For this review, take the finished solid that the model builds, in its own axes (mm). Face numbers are marked on the shaded views. A direction names the side the tool comes from. Coordinates: 2 decimals unless noted, no trailing zeros. Loops run counter-clockwise (first coordinate to the right, second up) from the corner with the lowest first, then second, coordinate; pieces in that order, holes last.
1. Take a section at A-A, the plane x = 23. State the section outline as (y, z) points, then the cut area to 3 significant figures.
2. Take a section at C-C, the plane y = 8. State the section outline as (x, z) points.
3. Machinability: for the marked faces 1, 2 and 3, which of the approach directions +Z, -Z, +X, -X, +Y, -Y give a long, thin tool a straight path to every point of the face, cutting with its end or side? Answer none if there is none.
4. Clearance check with flat-ended pins moving along their axes: P1, Ø1, axis at y = 19, z = 10, coming from the -X side; P2, Ø5.5, axis at x = -25, z = 7.5, coming from the +Y side; P3, Ø7, axis at x = -23, z = 10, coming from the +Y side. State where each tip first meets the part, or that it passes through.
5. Mouldability with a two-part tool opening along Z and no side actions: class the marked faces 4, 5 and 6 as pulls with the +Z half, pulls with the -Z half, needs draft (parallel to the pull), parting line crosses it, or undercut.
6. Take a section at D-D, the plane x = 0.5. State the section outline as (y, z) points.
7. Take a section at B-B, the plane z = 2.25. State the section outline as (x, y) points, then the cut area to 3 significant figures.
8. To check wall thickness, follow probe 1 along X at (y, z) = (-9, 9.25); probe 2 along X at (y, z) = (8.5, 8); probe 3 along X at (y, z) = (14.75, 10). State the ranges of each line that lie inside material, in increasing order.
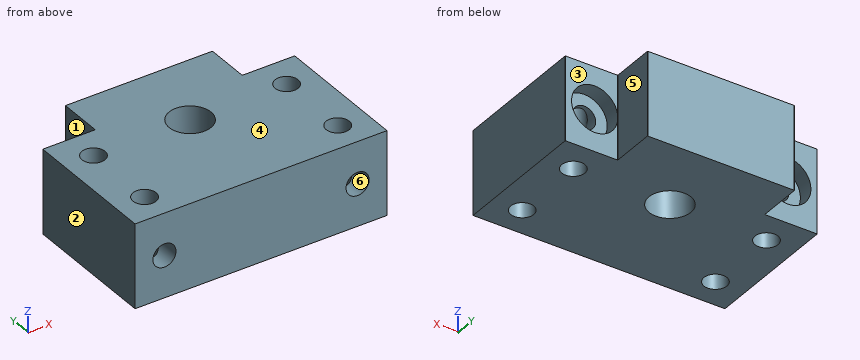
```python
from build123d import *

# Parameters (mm, degrees)
SKETCH_1_W                  = 60
SKETCH_1_H                  = 32.5
EXTRUDE_1_DEPTH             = 20
SKETCH_2_W                  = 35
SKETCH_2_H                  = 20
EXTRUDE_2_DEPTH             = 10.5
FILLET_1_R                  = 0.1
SKETCH_3_R                  = 5
SKETCH_3_R_2                = 2.75
CUT_EXTRUDE_1_DEPTH         = 45.895016427
HOLE_WIZARD_M5_1_AT_2_COUNT = 2
HOLE_WIZARD_M5_1_AT_2_PITCH = 46


with BuildPart() as part:
    # 스케치1 → 보스-돌출1 (new body)
    with BuildSketch(Plane.XY):
        Rectangle(SKETCH_1_W, SKETCH_1_H)
    extrude(amount=EXTRUDE_1_DEPTH)

    # 스케치2 → 보스-돌출2 (add)
    with BuildSketch(Plane(origin=(0, 16.25, 0), x_dir=(1, 0, 0), z_dir=(0, 1, 0))):
        with Locations((0, -10)):
            Rectangle(SKETCH_2_W, SKETCH_2_H)
    extrude(amount=EXTRUDE_2_DEPTH)

    # 필렛1
    fillet_1_edges = [part.edges().sort_by_distance(p)[0] for p in [
        (17.5, 16.25, 10),
        (-17.5, 16.25, 10),
        (17.5, 26.75, 10),
        (-17.5, 26.75, 10),
        (-30, 16.25, 10),
        (30, 16.25, 10),
    ]]
    fillet(fillet_1_edges, radius=FILLET_1_R)

    # 스케치3 → 컷-돌출1 (cut, through all)
    with BuildSketch(Plane.XY.offset(20)):
        with Locations((0, 8.75)):
            Circle(SKETCH_3_R)
        with Locations((-23, 8.75)):
            Circle(SKETCH_3_R_2)
        with Locations((-23, -9.25)):
            Circle(SKETCH_3_R_2)
        with Locations((23, 8.75)):
            Circle(SKETCH_3_R_2)
        with Locations((23, -9.25)):
            Circle(SKETCH_3_R_2)
    extrude(amount=-CUT_EXTRUDE_1_DEPTH, mode=Mode.SUBTRACT)

    # 스케치7 → M5 남비 머리 나사용 카운터보어1 (revolve, cut)
    with BuildSketch(Plane(origin=(23, 16.25, 10), x_dir=(0, 0, 1), z_dir=(1, 0, 0))):
        Polygon((0, 0), (0, 41.652366702), (2.75, 40), (2.75, 3.7), (5.5, 3.7), (5.5, 0), align=None)
    hole_wizard_m5_1 = revolve(axis=Axis((23, 22.6, 10), (0, -1, 0)), mode=Mode.SUBTRACT)

    # M5 남비 머리 나사용 카운터보어1 at 2: M5 남비 머리 나사용 카운터보어1 ×2
    with Locations(*[(-i * HOLE_WIZARD_M5_1_AT_2_PITCH, 0, 0) for i in range(1, HOLE_WIZARD_M5_1_AT_2_COUNT)]):
        add(hole_wizard_m5_1, mode=Mode.SUBTRACT)


solid = part.part
```
Results list:
1. outline: (-16.25, 0) - (-12, 0) - (-12, 7.25) - (-16.25, 7.25) - close; (-16.25, 12.75) - (-12, 12.75) - (-12, 20) - (-16.25, 20) - close; (-6.5, 0) - (6, 0) - (6, 7.25) - (-6.5, 7.25) - close; (-6.5, 12.75) - (6, 12.75) - (6, 20) - (-6.5, 20) - close; (11.5, 0) - (16.25, 0) - (16.25, 4.5) - (12.55, 4.5) - (12.55, 7.25) - (11.5, 7.25) - close; (11.5, 12.75) - (12.55, 12.75) - (12.55, 15.5) - (16.25, 15.5) - (16.25, 20) - (11.5, 20) - close
1. area: 291 mm2
2. outline: (-30, 0) - (-25.65, 0) - (-25.65, 9.25) arc R2.75 cw to (-25.65, 10.75) - (-25.65, 20) - (-30, 20) - close; (-20.35, 0) - (-4.94, 0) - (-4.94, 20) - (-20.35, 20) - (-20.35, 10.75) arc R2.75 cw to (-20.35, 9.25) - close; (4.94, 0) - (20.35, 0) - (20.35, 9.25) arc R2.75 cw to (20.35, 10.75) - (20.35, 20) - (4.94, 20) - close; (25.65, 0) - (30, 0) - (30, 20) - (25.65, 20) - (25.65, 10.75) arc R2.75 cw to (25.65, 9.25) - close
3. face 1: +Z, -Z, -X, +Y
3. face 2: +Z, -Z, -X, +Y, -Y
3. face 3: +Z, -Z, +X, +Y
4. P1: stops at x = -17.5
4. P2: stops at y = 16.25
4. P3: stops at y = 12.55
5. face 4: pulls with the +Z half
5. face 5: needs draft
5. face 6: undercut
6. outline: (-16.25, 0) - (3.78, 0) - (3.78, 20) - (-16.25, 20) - close; (13.72, 0) - (26.75, 0) - (26.75, 20) - (13.72, 20) - close
7. outline: (-30, -16.25) - (30, -16.25) - (30, 16.15) arc R0.1 ccw to (29.9, 16.25) - (17.6, 16.25) arc R0.1 cw to (17.5, 16.35) - (17.5, 26.65) arc R0.1 ccw to (17.4, 26.75) - (-17.4, 26.75) arc R0.1 ccw to (-17.5, 26.65) - (-17.5, 16.35) arc R0.1 cw to (-17.6, 16.25) - (-29.9, 16.25) arc R0.1 ccw to (-30, 16.15) - close; hole circle Ø5.5 at (-23, -9.25); hole circle Ø5.5 at (-23, 8.75); hole circle Ø10 at (0, 8.75); hole circle Ø5.5 at (23, -9.25); hole circle Ø5.5 at (23, 8.75)
7. area: 2,140 mm2
8. probe 1: x = -30 to -25.74, -20.26 to 20.26, 25.74 to 30
8. probe 2: x = -30 to -25.74, -20.26 to -4.99, 4.99 to 20.26, 25.74 to 30
8. probe 3: x = -30 to -28.5, -17.5 to 17.5, 28.5 to 30
